Verification items for this drawing (mm, ordinates from the low corner). A direction names the side the tool comes from. Give positions to 0.01 mm unless a question says otherwise; leave off trailing zeros. Write each loop counter-clockwise with the first axis right and the second up, starting at its lowest first coordinate (ties: lowest second). Pieces come first, ordered by that corner, then holes. Notation, with made-up numbers: (-4.5, 23.25) -> (27.5, 23.25) arc R7 ccw to (27.5, 36.25) -> close; hole circle Ø2 at (5.25, 82). An arc over 180 degrees is marked (long way). Use one line per item in the form item = value. Start each with the question number.
(1) Scan lines: L1, parallel to Y at x = 34.5, z = 13.5; L2, parallel to Z at x = 75.5, y = 59.5; L3, parallel to Y at x = 36, z = 41. Record each from-to range of solid material in increasing order.
(2) Section check D-D, the plane z = 27. Record the cut outline in (x, y), plus the area to 3 significant figures.
(3) Section check B-B, the plane x = 51. Record the cut outline in (y, z) (1 decimal), plus the area to 3 significant figures.
(4) Section check A-A, the plane y = 41. Record the cut outline in (x, z) (1 decimal), plus the area to 3 significant figures.
(5) Release check for a two-part mould opening along X. For the marked faces 1, 2 and 3 record: pulls with the +X half, pulls with the -X half, needs draft (parallel to the pull), parting line crosses it, or undercut.
(6) Section check C-C, the plane x = 29. Record the cut outline in (y, z).
(7) Set-up check for the marked faces 4 and 5: record each of +Z, -Z, +X, -X, +Y, -Y from which the full face is reachable in a straight line by a thin tool's end or side.
(8) Depth check by flat-ended pin: pin 1 Ø5 at (x, z) = (55.5, 12.5) entering from -Y; pin 2 Ø12 at (x, z) = (21, 28.5) entering from +Y (1 decimal); pin 3 Ø12 at (x, y) = (46.5, 52) entering from -Z. Enter the tip coordinate at first touch or a pass-through.
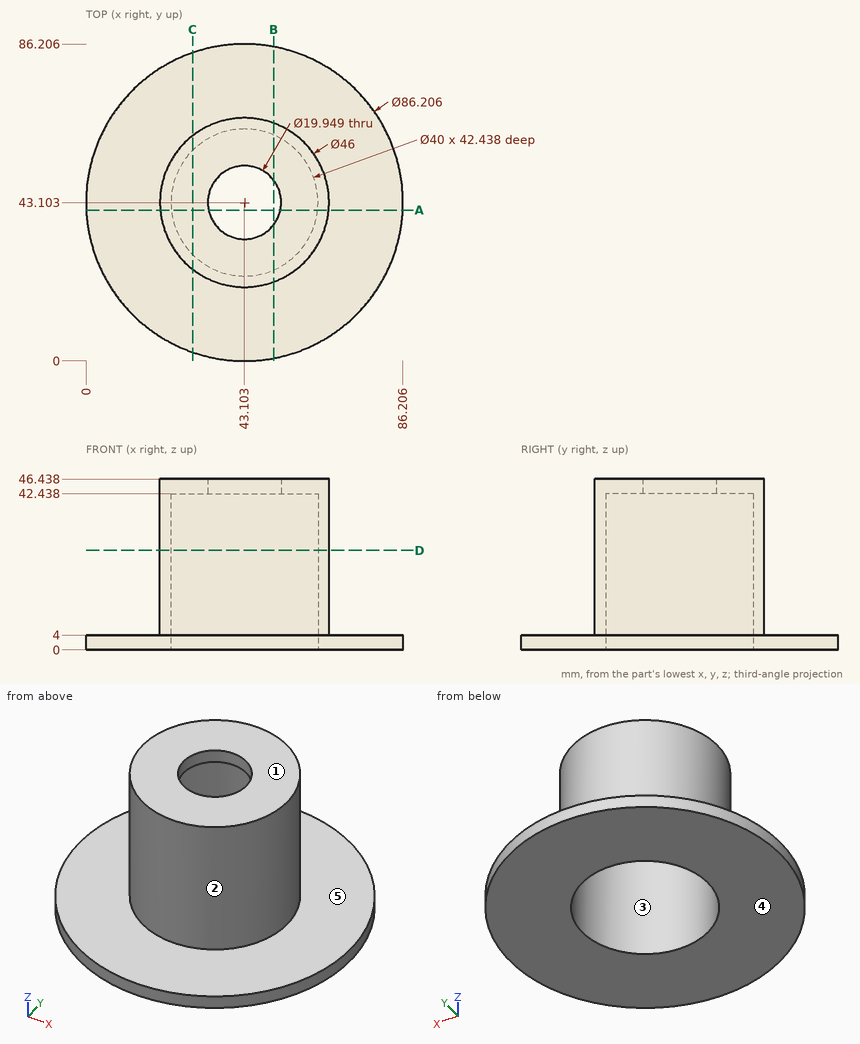
Completed:
q1.L1 = 21.77 to 25.05, 61.16 to 64.43
q1.L2 = 0 to 4
q1.L3 = 21.23 to 24.41, 61.8 to 64.98
q2.outline = circle Ø46 at (43.1, 43.1); hole circle Ø40 at (43.1, 43.1)
q2.area = 405 mm²
q3.outline = (0.7, 0) -> (24.7, 0) -> (24.7, 42.4) -> (37, 42.4) -> (37, 46.4) -> (21.5, 46.4) -> (21.5, 4) -> (0.7, 4) -> close; (49.2, 42.4) -> (61.5, 42.4) -> (61.5, 0) -> (85.5, 0) -> (85.5, 4) -> (64.7, 4) -> (64.7, 46.4) -> (49.2, 46.4) -> close
q3.area = 564 mm²
q4.outline = (0.1, 0) -> (23.2, 0) -> (23.2, 42.4) -> (33.4, 42.4) -> (33.4, 46.4) -> (20.2, 46.4) -> (20.2, 4) -> (0.1, 4) -> close; (52.9, 42.4) -> (63, 42.4) -> (63, 0) -> (86.2, 0) -> (86.2, 4) -> (66, 4) -> (66, 46.4) -> (52.9, 46.4) -> close
q4.area = 522 mm²
q5.face_1 = needs draft
q5.face_2 = parting line crosses it
q5.face_3 = undercut
q6.outline = (2.37, 0) -> (28.92, 0) -> (28.92, 42.44) -> (57.28, 42.44) -> (57.28, 0) -> (83.83, 0) -> (83.83, 4) -> (61.27, 4) -> (61.27, 46.44) -> (24.93, 46.44) -> (24.93, 4) -> (2.37, 4) -> close
q7.face_4 = -Z, +X, -X, +Y, -Y
q7.face_5 = +Z
q8.pin_1 = 22.34
q8.pin_2 = 59.5
q8.pin_3 = 42.44
